```python
from build123d import *

# Parameters (mm, degrees)
SCHIZZO1_W               = 220
SCHIZZO1_H               = 220
SCHIZZO1_R               = 4
BASE_FLANGIA1_DEPTH      = 3
SCHIZZO2_R               = 4
TAGLIO_ESTRUSIONE1_DEPTH = 156.592416268


# Sheet-metal steps are written as plain solids
with BuildPart() as part:
    # Schizzo1 → Base-Flangia1 (new body)
    with BuildSketch(Plane.XY):
        Rectangle(SCHIZZO1_W, SCHIZZO1_H)
        with Locations((0, 100)):
            Circle(SCHIZZO1_R, mode=Mode.SUBTRACT)
        with Locations((86.602540378, 50)):
            Circle(SCHIZZO1_R, mode=Mode.SUBTRACT)
        with Locations((86.602540378, -50)):
            Circle(SCHIZZO1_R, mode=Mode.SUBTRACT)
        with Locations((0, -100)):
            Circle(SCHIZZO1_R, mode=Mode.SUBTRACT)
        with Locations((-86.602540378, -50)):
            Circle(SCHIZZO1_R, mode=Mode.SUBTRACT)
        with Locations((-86.602540378, 50)):
            Circle(SCHIZZO1_R, mode=Mode.SUBTRACT)
    extrude(amount=-BASE_FLANGIA1_DEPTH)

    # Schizzo2 → Taglio-Estrusione1 (cut, through all)
    with BuildSketch(Plane.XY):
        with Locations((-19.75, -44)):
            Circle(SCHIZZO2_R)
        with Locations((-44, -19.75)):
            Circle(SCHIZZO2_R)
        with Locations((-44, 34)):
            Circle(SCHIZZO2_R)
        with Locations((34, -44)):
            Circle(SCHIZZO2_R)
    extrude(amount=-TAGLIO_ESTRUSIONE1_DEPTH, mode=Mode.SUBTRACT)


solid = part.part
```
For this review, take the finished solid that the model builds, in its own axes (mm). Coordinates: 2 decimals unless noted, no trailing zeros. Loops run counter-clockwise (first coordinate to the right, second up) from the corner with the lowest first, then second, coordinate; pieces in that order, holes last.
1. Mouldability with a two-part tool opening along X and no side actions: class faces 1 (the flat face through (-2, 2, 0)), 2 (the cylindrical face through (1.846, 96.451, -1.479)), 3 (the cylindrical face through (-82.908, 48.468, -1.479)) as +X half, -X half, draft (parallel to the pull), parting line (faces both ways), or undercut.
2. Insertion check: P1, Ø5, axis at x = 34, y = -44, coming from the -Z side. The pin has a flat end and moves straight along its axis. Give the tip position at first contact, or say it passes through.
3. Add section A-A, the plane x = -19.75. Give the boundary of the cut face in (y, z).
4. Add section C-C, the plane x = -44. Give the boundary of the cut face in (y, z).
5. Add section D-D, the plane x = -88. Give the boundary of the cut face in (y, z), then the cut area to 3 significant figures.
6. For line 1 (X direction, y = -44.5, z = -0.6); line 2 (Y direction, x = -87, z = -1.1), list the stretches that pass through material, from the lowest coordinate up.
Result:
1. face 1: draft
1. face 2: undercut
1. face 3: undercut
2. P1: passes through
3. outline: (-110, -3) - (-48, -3) - (-48, 0) - (-110, 0) - close; (-40, -3) - (110, -3) - (110, 0) - (-40, 0) - close
4. outline: (-110, -3) - (-23.75, -3) - (-23.75, 0) - (-110, 0) - close; (-15.75, -3) - (30, -3) - (30, 0) - (-15.75, 0) - close; (38, -3) - (110, -3) - (110, 0) - (38, 0) - close
5. outline: (-110, -3) - (-53.75, -3) - (-53.75, 0) - (-110, 0) - close; (-46.25, -3) - (46.25, -3) - (46.25, 0) - (-46.25, 0) - close; (53.75, -3) - (110, -3) - (110, 0) - (53.75, 0) - close
5. area: 615 mm2
6. line 1: x = -110 to -23.72, -15.78 to 30.03, 37.97 to 110
6. line 2: y = -110 to -53.98, -46.02 to 46.02, 53.98 to 110
